from build123d import *

# Parameters (mm, degrees)
SKETCH1_W            = 297
SKETCH1_H            = 100
BASE_FLANGE1_DEPTH   = 2
EDGE_FLANGE1_START   = -50
EDGE_FLANGE1_DEPTH   = 100
EDGE_FLANGE1_2_DEPTH = 100


# Read off the part's stored shape, not the designer's step: Edge-Flange1
# Sheet-metal steps are written as plain solids
with BuildPart() as part:
    # Sketch1 → Base-Flange1 (new body)
    with BuildSketch(Plane(origin=(0, 0, 0), x_dir=(1, 0, 0), z_dir=(0, 1, 0))):
        Rectangle(SKETCH1_W, SKETCH1_H)
    extrude(amount=-BASE_FLANGE1_DEPTH)

    # Edge-Flange1 outline → Edge-Flange1 (cut)
    with BuildSketch(Plane.XY.offset(EDGE_FLANGE1_START)):
        with BuildLine():
            ThreePointArc((-145.721040868, -2), (-147.375308077, -1.443395312), (-148.356643266, 0))
            Line((-148.356643266, 0), (-148.5, 0))
            Line((-148.5, 0), (-148.5, -2))
            Line((-148.5, -2), (-145.721040868, -2))
        make_face()
    extrude(amount=EDGE_FLANGE1_DEPTH, mode=Mode.SUBTRACT)

    # Edge-Flange1 2 outline → Edge-Flange1 2 (add)
    with BuildSketch(Plane.XY.offset(EDGE_FLANGE1_START)):
        with BuildLine():
            Line((-147.662768346, 15.975331626), (-148.453890453, 0.879822578))
            ThreePointArc((-148.453890453, 0.879822578), (-148.441075999, 0.435953289), (-148.356643266, 0))
            Line((-148.356643266, 0), (-145.721040868, 0))
            ThreePointArc((-145.721040868, 0), (-146.255351629, 0.22955802), (-146.456631383, 0.775150665))
            Line((-146.456631383, 0.775150665), (-145.665509277, 15.870659713))
            Line((-145.665509277, 15.870659713), (-147.662768346, 15.975331626))
        make_face()
    extrude(amount=EDGE_FLANGE1_2_DEPTH)


solid = part.part
The listing builds one solid part. Answer for the finished solid, in the listing's coordinates (mm). Round coordinates to 2 decimals unless told otherwise and drop trailing zeros. Loops run counter-clockwise (first coordinate to the right, second up) from the corner with the lowest first, then second, coordinate; pieces in that order, holes last. Notation, with made-up numbers: M 59,-19.5 L 85,-19.5 A18 cw 85,3.5 Z; hole C -16,29.5 d2. An arc over 180 degrees is marked long. Return JSON: item names as keys, results as strings.
Q1. Find the intervals of material crossed by line 1 along Y through (x, z) = (60.5, 29); line 2 along X through (y, z) = (9.25, 7); line 3 along X through (y, z) = (3, -18), in increasing order. Write a range as from..to.
Results list:
{"line 1": "y = -2..0", "line 2": "x = -148.02..-146.01", "line 3": "x = -148.34..-146.34"}
Q2. The mould has two halves that part along Y. Classify faces 1 (the face through (-1, 0, -1)), 2 (the face through (-1, -1, 50)), 3 (the face through (-146.067, 8.217, -0.7)): released by +Y, released by -Y, zero draft, split by the parting line, or undercut.
Results list:
{"face 1": "released by +Y", "face 2": "zero draft", "face 3": "undercut"}
Q3. Find section A-A, the plane z = -39.5. Determine the outline of the cut face in (x, y).
Results list:
{"outline": "M -148.45,0.88 A2.74 ccw -145.72,-2 L 148.5,-2 L 148.5,0 L -145.72,0 A0.74 cw -146.46,0.78 L -145.67,15.87 L -147.66,15.98 Z"}
Q4. Find section B-B, the plane x = -102. Determine the outline of the cut face in (y, z).
Results list:
{"outline": "M -2,-50 L 0,-50 L 0,50 L -2,50 Z"}
Q5. Find section C-C, the plane y = 7.25. Determine the outline of the cut face in (x, z).
Results list:
{"outline": "M -148.12,-50 L -146.12,-50 L -146.12,50 L -148.12,50 Z"}
Q6. Each of these flat-tipped pins is pushed along its axis until it touches: pin 1 Ø5 at (y, z) = (12.5, -21.5) entering from +X; pin 2 Ø1 at (y, z) = (0, -27) entering from -X. Where does it stop, or does it pass through?
Results list:
{"pin 1": "stops at x = -145.71", "pin 2": "stops at x = -148.45"}
